Design review of the part built by this model. Coordinates are the model's own, in mm. Face numbers are marked on the shaded views. A direction names the side the tool comes from. Coordinates: 2 decimals unless noted, no trailing zeros. Loops run counter-clockwise (first coordinate to the right, second up) from the corner with the lowest first, then second, coordinate; pieces in that order, holes last.
from build123d import *

# Parameters (mm, degrees)
F1_DEPTH = 30
F3_DEPTH = 8.001
F4_R     = 1
F6_DEPTH = 3
F8_DEPTH = 25
F9_R     = 2


with BuildPart() as f1:
    # F0 (on Top) → F1 (new body)
    with BuildSketch(Plane.XY):
        Polygon((8, 0), (8, 36), (4.5, 36), (4.5, 30), (0, 30), (0, 0), align=None)
    extrude(amount=F1_DEPTH)

    # F2 (on face) → F3 (cut, through all)
    with BuildSketch(Plane(origin=(0, 0, 0), x_dir=(0, -1, 0), z_dir=(-1, 0, 0))):
        with BuildLine():
            ThreePointArc((-7.194215, 20.5), (-5.780001, 21.085786), (-5.194215, 22.5))
            ThreePointArc((-5.194215, 22.5), (-5.780001, 23.914214), (-7.194215, 24.5))
            ThreePointArc((-7.194215, 24.5), (-9.194215, 22.5), (-7.194215, 20.5))
        make_face()
        with BuildLine():
            ThreePointArc((-7.194215, 20.5), (-9.194215, 22.5), (-7.194215, 24.5))
            Line((-7.194215, 24.5), (-15, 24.5))
            Line((-15, 24.5), (-22.805785, 24.5))
            ThreePointArc((-22.805785, 24.5), (-21.391572, 23.914214), (-20.805785, 22.5))
            ThreePointArc((-20.805785, 22.5), (-21.391572, 21.085786), (-22.805785, 20.5))
            Line((-22.805785, 20.5), (-15, 20.5))
            Line((-15, 20.5), (-7.194215, 20.5))
        make_face()
        with BuildLine():
            ThreePointArc((-20.805785, 22.5), (-21.391572, 23.914214), (-22.805785, 24.5))
            ThreePointArc((-22.805785, 24.5), (-24.805785, 22.5), (-22.805785, 20.5))
            ThreePointArc((-22.805785, 20.5), (-21.391572, 21.085786), (-20.805785, 22.5))
        make_face()
        with BuildLine():
            ThreePointArc((-7.194215, 5.5), (-5.780001, 6.085786), (-5.194215, 7.5))
            ThreePointArc((-5.194215, 7.5), (-5.780001, 8.914214), (-7.194215, 9.5))
            ThreePointArc((-7.194215, 9.5), (-9.194215, 7.5), (-7.194215, 5.5))
        make_face()
        with BuildLine():
            ThreePointArc((-7.194215, 5.5), (-9.194215, 7.5), (-7.194215, 9.5))
            Line((-7.194215, 9.5), (-15, 9.5))
            Line((-15, 9.5), (-22.805785, 9.5))
            ThreePointArc((-22.805785, 9.5), (-21.391572, 8.914214), (-20.805785, 7.5))
            ThreePointArc((-20.805785, 7.5), (-21.391572, 6.085786), (-22.805785, 5.5))
            Line((-22.805785, 5.5), (-15, 5.5))
            Line((-15, 5.5), (-7.194215, 5.5))
        make_face()
        with BuildLine():
            ThreePointArc((-20.805785, 7.5), (-21.391572, 8.914214), (-22.805785, 9.5))
            ThreePointArc((-22.805785, 9.5), (-24.805785, 7.5), (-22.805785, 5.5))
            ThreePointArc((-22.805785, 5.5), (-21.391572, 6.085786), (-20.805785, 7.5))
        make_face()
    extrude(amount=-F3_DEPTH, mode=Mode.SUBTRACT)

    # F4
    f4_edges = [f1.edges().sort_by_distance(p)[0] for p in [
        (4.5, 36, 15),
        (8, 36, 15),
    ]]
    fillet(f4_edges, radius=F4_R)

    # F5 (on face) → F6 (cut)
    with BuildSketch(Plane.YZ.offset(8)):
        with BuildLine():
            ThreePointArc((7.194215, 18.25), (10.199419, 19.494796), (11.444215, 22.5))
            ThreePointArc((11.444215, 22.5), (10.199419, 25.505204), (7.194215, 26.75))
            ThreePointArc((7.194215, 26.75), (2.944215, 22.5), (7.194215, 18.25))
        make_face()
        with BuildLine():
            ThreePointArc((7.194215, 26.75), (10.199419, 25.505204), (11.444215, 22.5))
            ThreePointArc((11.444215, 22.5), (10.199419, 19.494796), (7.194215, 18.25))
            Line((7.194215, 18.25), (22.805785, 18.25))
            ThreePointArc((22.805785, 18.25), (18.555785, 22.5), (22.805785, 26.75))
            Line((22.805785, 26.75), (7.194215, 26.75))
        make_face()
        with BuildLine():
            ThreePointArc((27.055785, 22.5), (25.810989, 25.505204), (22.805785, 26.75))
            ThreePointArc((22.805785, 26.75), (18.555785, 22.5), (22.805785, 18.25))
            ThreePointArc((22.805785, 18.25), (25.810989, 19.494796), (27.055785, 22.5))
        make_face()
        with BuildLine():
            ThreePointArc((7.194215, 3.25), (10.199419, 4.494796), (11.444215, 7.5))
            ThreePointArc((11.444215, 7.5), (10.199419, 10.505204), (7.194215, 11.75))
            ThreePointArc((7.194215, 11.75), (2.944215, 7.5), (7.194215, 3.25))
        make_face()
        with BuildLine():
            ThreePointArc((7.194215, 11.75), (10.199419, 10.505204), (11.444215, 7.5))
            ThreePointArc((11.444215, 7.5), (10.199419, 4.494796), (7.194215, 3.25))
            Line((7.194215, 3.25), (22.805785, 3.25))
            ThreePointArc((22.805785, 3.25), (18.555785, 7.5), (22.805785, 11.75))
            Line((22.805785, 11.75), (7.194215, 11.75))
        make_face()
        with BuildLine():
            ThreePointArc((27.055785, 7.5), (25.810989, 10.505204), (22.805785, 11.75))
            ThreePointArc((22.805785, 11.75), (18.555785, 7.5), (22.805785, 3.25))
            ThreePointArc((22.805785, 3.25), (25.810989, 4.494796), (27.055785, 7.5))
        make_face()
    extrude(amount=-F6_DEPTH, mode=Mode.SUBTRACT)

    # F7 (on face) → F8 (join)
    with BuildSketch(Plane(origin=(0, 0, 0), x_dir=(0, -1, 0), z_dir=(-1, 0, 0))):
        Polygon((-18.8505, 12.5), (-11.865322, 12.5), (-11.865322, 15), (-11.865322, 17.5), (-18.8505, 17.5), (-18.8505, 15), align=None)
    extrude(amount=F8_DEPTH)

    # F9
    f9_edges = [f1.edges().sort_by_distance(p)[0] for p in [
        (0, 18.8505, 15),
        (0, 15.357911, 17.5),
        (0, 15.357911, 12.5),
        (0, 11.865322, 15),
        (-12.5, 11.865322, 12.5),
        (-12.5, 11.865322, 17.5),
        (-12.5, 18.8505, 12.5),
        (-12.5, 18.8505, 17.5),
    ]]
    fillet(f9_edges, radius=F9_R)


solid = f1.part
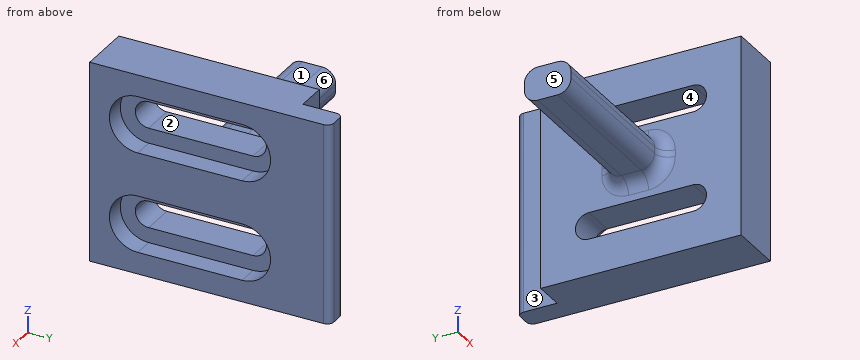
Q1. Take a section at C-C, the plane z = 27.25. Write out the cut boundary in (x, y), then the cut area to 3 significant figures.
Q2. Take a section at A-A, the plane z = 23.75. Write out the cut boundary in (x, y), then the cut area to 3 significant figures.
Q3. Take a section at D-D, the plane x = -16. Write out the cut boundary in (y, z), then the cut area to 3 significant figures.
Q4. The part is to be moulded in two halves that separate along Y. For the marked faces 4, 5 and 6, say which applies: pulls with the +Y half, pulls with the -Y half, needs draft (parallel to the pull), parting line crosses it, or undercut.
Q5. Clearance check with flat-ended pins moving along their axes: pin 1 Ø3.5 at (x, y) = (-16.5, 15.5) entering from +Z; pin 2 Ø5 at (y, z) = (8.5, 11.5) entering from -X; pin 3 Ø1.5 at (y, z) = (31.5, 17) entering from -X. State where each tip first meets the part, or that it passes through.
Q6. Take a section at B-B, the plane y = 6. Write out the cut boundary in (x, z), then the cut area to 3 significant figures.
Q7. For line 1 (Z direction, x = 6.5, y = 22); line 2 (Y direction, x = 1.5, z = 22.5); line 3 (X direction, y = 5, z = 17.75), list the stretches that pass through material, from the lowest coordinate up.
Q8. Machinability: for the marked faces 1, 2 and 3, which of the approach directions +Z, -Z, +X, -X, +Y, -Y give a long, thin tool a straight path to every point of the face, cutting with its end or side? Answer none if there is none.
Entries:
1. outline: (0, 0) - (8, 0) - (8, 35) arc R1 ccw to (7, 36) - (5.5, 36) arc R1 ccw to (4.5, 35) - (4.5, 30) - (0, 30) - close
1. area: 261 mm2
2. outline: (0, 0) - (8, 0) - (8, 3.13) - (5, 3.13) - (5, 5.63) - (0, 5.63) - close; (0, 24.37) - (5, 24.37) - (5, 26.87) - (8, 26.87) - (8, 35) arc R1 ccw to (7, 36) - (5.5, 36) arc R1 ccw to (4.5, 35) - (4.5, 30) - (0, 30) - close
2. area: 95.7 mm2
3. outline: (11.87, 14.5) arc R2 ccw to (13.87, 12.5) - (16.85, 12.5) arc R2 ccw to (18.85, 14.5) - (18.85, 15.5) arc R2 ccw to (16.85, 17.5) - (13.87, 17.5) arc R2 ccw to (11.87, 15.5) - close
3. area: 31.5 mm2
4. face 4: undercut
4. face 5: needs draft
4. face 6: pulls with the +Y half
5. pin 1: stops at z = 17.5
5. pin 2: stops at x = -0.03
5. pin 3: stops at x = 4.5
6. outline: (0, 0) - (8, 0) - (8, 3.42) - (5, 3.42) - (5, 5.9) - (0, 5.9) - close; (0, 9.1) - (5, 9.1) - (5, 11.58) - (8, 11.58) - (8, 18.42) - (5, 18.42) - (5, 20.9) - (0, 20.9) - close; (0, 24.1) - (5, 24.1) - (5, 26.58) - (8, 26.58) - (8, 30) - (0, 30) - close
6. area: 159 mm2
7. line 1: z = 0 to 3.25, 11.75 to 18.25, 26.75 to 30
7. line 2: y = 0 to 5.19, 24.81 to 30
7. line 3: x = 0 to 8
8. face 1: +Z, -X, +Y, -Y
8. face 2: +X, -X
8. face 3: +Z, -Z, -X, +Y
